from build123d import *

# Parameters (mm, degrees)
F1_DEPTH      = 58
F3_DEPTH      = 58.001
F4_W          = 36
F4_H          = 6.6
F5_DEPTH      = 127
F5_DEPTH_BACK = 127
F7_DEPTH      = 29.001
F8_R          = 3
F9_DEPTH      = 25


with BuildPart() as f1:
    # F0 (on Front) → F1 (new body)
    with BuildSketch(Plane.XZ):
        with BuildLine():
            ThreePointArc((-60.907962, 9), (-61.979652, 4.556598), (-62.339865, 0))
            Line((-62.339865, 0), (-51.339865, 0))
            Line((-51.339865, 0), (-51.339865, 9))
            Line((-51.339865, 9), (-60.907962, 9))
        make_face()
        with BuildLine():
            ThreePointArc((-33.339865, 29), (-50.369251, 23.473389), (-60.907962, 9))
            Line((-60.907962, 9), (-51.339865, 9))
            Line((-51.339865, 9), (-51.339865, 0))
            Line((-51.339865, 0), (53.660135, 0))
            Line((53.660135, 0), (53.660135, 9))
            Line((53.660135, 9), (63.228233, 9))
            ThreePointArc((63.228233, 9), (52.689522, 23.473389), (35.660135, 29))
            Line((35.660135, 29), (-33.339865, 29))
        make_face()
        with BuildLine():
            Line((53.660135, 9), (53.660135, 0))
            Line((53.660135, 0), (64.660135, 0))
            ThreePointArc((64.660135, 0), (64.299923, 4.556598), (63.228233, 9))
            Line((63.228233, 9), (53.660135, 9))
        make_face()
    extrude(amount=F1_DEPTH)

    # F2 (on face) → F3 (cut, through all)
    with BuildSketch(Plane.XZ.offset(58)):
        with BuildLine():
            Line((-62.339865, 0), (-51.339865, 0))
            Line((-51.339865, 0), (-51.339865, 9))
            Line((-51.339865, 9), (-60.907962, 9))
            ThreePointArc((-60.907962, 9), (-61.979652, 4.556598), (-62.339865, 0))
        make_face()
        with BuildLine():
            Line((53.660135, 9), (53.660135, 0))
            Line((53.660135, 0), (64.660135, 0))
            ThreePointArc((64.660135, 0), (64.299923, 4.556598), (63.228233, 9))
            Line((63.228233, 9), (53.660135, 9))
        make_face()
    extrude(amount=-F3_DEPTH, mode=Mode.SUBTRACT)

    # F4 (on Right) → F5 (cut, two sides)
    with BuildSketch(Plane.YZ) as f5_sk:
        with Locations((-29, 25.7)):
            Rectangle(F4_W, F4_H)
    extrude(amount=F5_DEPTH, mode=Mode.SUBTRACT)
    extrude(f5_sk.sketch, amount=-F5_DEPTH_BACK, mode=Mode.SUBTRACT)

    # F6 (on face) → F7 (cut, through all)
    with BuildSketch(Plane(origin=(0, 0, 0), x_dir=(1, 0, 0), z_dir=(0, 0, -1))):
        with BuildLine():
            ThreePointArc((-37.339865, 35.5), (-43.839865, 29), (-37.339865, 22.5))
            Line((-37.339865, 22.5), (-18.339865, 22.5))
            ThreePointArc((-18.339865, 22.5), (-11.839865, 29), (-18.339865, 35.5))
            Line((-18.339865, 35.5), (-37.339865, 35.5))
        make_face()
        with BuildLine():
            ThreePointArc((20.660135, 35.611376), (14.160135, 29.111376), (20.660135, 22.611376))
            Line((20.660135, 22.611376), (39.660135, 22.611376))
            ThreePointArc((39.660135, 22.611376), (46.160135, 29.111376), (39.660135, 35.611376))
            Line((39.660135, 35.611376), (20.660135, 35.611376))
        make_face()
    extrude(amount=-F7_DEPTH, mode=Mode.SUBTRACT)

    # F8
    f8_edges = [f1.edges().sort_by_distance(p)[0] for p in [
        (1.160135, -58, 29),
        (1.160135, 0, 29),
    ]]
    fillet(f8_edges, radius=F8_R)

    # F6 (on face) → F9 (cut)
    with BuildSketch(Plane(origin=(0, 0, 0), x_dir=(1, 0, 0), z_dir=(0, 0, -1))):
        with BuildLine():
            ThreePointArc((-37.339865, 35.5), (-43.839865, 29), (-37.339865, 22.5))
            Line((-37.339865, 22.5), (-18.339865, 22.5))
            ThreePointArc((-18.339865, 22.5), (-11.839865, 29), (-18.339865, 35.5))
            Line((-18.339865, 35.5), (-37.339865, 35.5))
        make_face()
        with BuildLine():
            ThreePointArc((20.660135, 35.611376), (14.160135, 29.111376), (20.660135, 22.611376))
            Line((20.660135, 22.611376), (39.660135, 22.611376))
            ThreePointArc((39.660135, 22.611376), (46.160135, 29.111376), (39.660135, 35.611376))
            Line((39.660135, 35.611376), (20.660135, 35.611376))
        make_face()
    extrude(amount=F9_DEPTH, mode=Mode.SUBTRACT)


solid = f1.part
Input: part model. Units: mm. Frame: model coordinates. A direction names the side the tool comes from. Coordinates: 2 decimals unless noted, no trailing zeros. Order: outer loops, then holes, each group sorted by start corner. A loop starts at its lowest first (then second) coordinate and runs counter-clockwise, first axis right, second up. Notation, with made-up numbers: M 64.5,60 L 78.5,60 A25 ccw 78.5,92 Z; hole C 53,71.25 d6. An arc over 180 degrees is marked long. Write item = value, one per line. Start each with the question number.
(1) Line query: line 1 along Y through (x, z) = (-22, 10.5); line 2 along Y through (x, z) = (28, 12.25); line 3 along X through (y, z) = (-54.5, 5.25). Output: solid intervals per line, ascending. Write a range as [from, to].
(2) First-contact query: P1, Ø2, axis at y = -19.5, z = 12, coming from the -X side; P2, Ø12, axis at y = -20, z = 22, coming from the -X side; P3, Ø4, axis at y = -18.5, z = 12, coming from the +X side. Flat tips, straight axial feed; report the tip coordinate or a pass-through.
(3) Reachability of faces 1 (the flat face through (30, -35.611, 11)), 2 (the flat face through (53.66, -29, 5)), 3 (the flat face through (2, -47, 26)) from +Z, -Z, +X, -X, +Y, -Y: full face, straight path, thin tool, end or side. Return the list, or none.
(4) Pull-direction query (Y, two-part tool) for faces 4 (the cylindrical face through (0.68, -0.86, 28.1)), 5 (the flat face through (-51.34, -29, 4)), 6 (the flat face through (2, -11, 26)), 7 (the flat face through (0, -58, 13)); classes: released by +Y, released by -Y, zero draft, split by the parting line, or undercut.
(5) Section B-B on y = -45.5. Output: boundary loops of the cut face in (x, z).
(6) Section A-A on y = -30. Output: boundary loops of the cut face in (x, z).
(7) Section C-C on z = 17.25. Give the number of separate pieces and of enclosed holes in the cut face, and give its area (3 significant figures).
Result set:
q1.line_1 = [-58, -35.5], [-22.5, 0]
q1.line_2 = [-58, -35.61], [-22.61, 0]
q1.line_3 = [-51.34, 53.66]
q2.P1 = -60.17
q2.P2 = -57.53
q2.P3 = 62.88
q3.face_1 = +Z, -Z
q3.face_2 = -Z, +X, +Y, -Y
q3.face_3 = +Z, +X, -X
q4.face_4 = released by +Y
q4.face_5 = zero draft
q4.face_6 = undercut
q4.face_7 = released by -Y
q5.outline = M -60.91,9 L -51.34,9 L -51.34,0 L 53.66,0 L 53.66,9 L 63.23,9 A29 ccw 54.08,22.4 L -51.76,22.4 A29 ccw Z
q6.outline = M -60.91,9 L -51.34,9 L -51.34,0 L -43.76,0 L -43.76,22.4 L -51.76,22.4 A29 ccw Z; M -11.92,0 L 14.22,0 L 14.22,22.4 L -11.92,22.4 Z; M 46.1,0 L 53.66,0 L 53.66,9 L 63.23,9 A29 ccw 54.08,22.4 L 46.1,22.4 Z
q7.separate_pieces = 1
q7.enclosed_holes = 2
q7.area = 5,940 mm²
